```python
from build123d import *

# Parameters (mm, degrees)
EXTRUDE_1_DEPTH = 50


with BuildPart() as part:
    # 草图1 → 凸台-拉伸1 (new body)
    with BuildSketch(Plane.XY):
        with BuildLine():
            Line((-3.068719851, 0.075307347), (-3.068719851, 3.975307347))
            Line((-3.068719851, 3.975307347), (-4.918719851, 3.975307347))
            Line((-4.918719851, 3.975307347), (-4.918719851, 3.125307347))
            Line((-4.918719851, 3.125307347), (-3.918719851, 3.125307347))
            Line((-3.918719851, 3.125307347), (-3.918719851, -3.824692653))
            ThreePointArc((-3.918719851, -3.824692653), (-3.420801379, -5.026774181), (-2.218719851, -5.524692653))
            Line((-2.218719851, -5.524692653), (3.081280149, -5.524692653))
            ThreePointArc((3.081280149, -5.524692653), (4.283361677, -5.026774181), (4.781280149, -3.824692653))
            Line((4.781280149, -3.824692653), (4.781280149, 3.125307347))
            Line((4.781280149, 3.125307347), (5.781280149, 3.125307347))
            Line((5.781280149, 3.125307347), (5.781280149, 3.975307347))
            Line((5.781280149, 3.975307347), (3.931280149, 3.975307347))
            Line((3.931280149, 3.975307347), (3.931280149, 0.075307347))
            Line((3.931280149, 0.075307347), (1.809959806, -2.046012996))
            Line((1.809959806, -2.046012996), (2.110480188, -2.346533378))
            Line((2.110480188, -2.346533378), (3.931280149, -1.126774181))
            Line((3.931280149, -1.126774181), (3.931280149, -3.824692653))
            ThreePointArc((3.931280149, -3.824692653), (3.682320913, -4.425733417), (3.081280149, -4.674692653))
            Line((3.081280149, -4.674692653), (-2.218719851, -4.674692653))
            ThreePointArc((-2.218719851, -4.674692653), (-2.819760615, -4.425733417), (-3.068719851, -3.824692653))
            Line((-3.068719851, -3.824692653), (-3.068719851, -1.126774181))
            Line((-3.068719851, -1.126774181), (-1.247919889, -2.346533378))
            Line((-1.247919889, -2.346533378), (-0.947399507, -2.046012996))
            Line((-0.947399507, -2.046012996), (-3.068719851, 0.075307347))
        make_face()
    extrude(amount=EXTRUDE_1_DEPTH)


solid = part.part
```
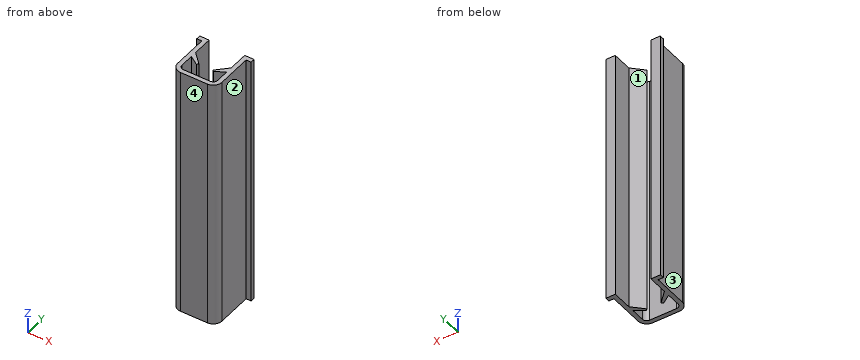
Part model, mm, in its own coordinate system. Face numbers are marked on the shaded views. Round coordinates to 2 decimals unless told otherwise and drop trailing zeros. Write each loop counter-clockwise with the first axis right and the second up, starting at its lowest first coordinate (ties: lowest second). Pieces come first, ordered by that corner, then holes. Notation, with made-up numbers: M 45.25,62 L 76.25,62 A27 ccw 76.25,94 Z; hole C 87.25,36.5 d2. An arc over 180 degrees is marked long. One line per question, with ' | ' between items.
(1) Two-plate mould, pull along X, no slides. Class the marked faces 1, 2, 3 and 4: released by +X, released by -X, zero draft, split by the parting line, or undercut.
Answer key:
face 1: undercut | face 2: released by +X | face 3: released by -X | face 4: zero draft
(2) Probe line 1 along X through (y, z) = (3.25, 38); line 2 along X through (y, z) = (-3.75, 35.5); line 3 along X through (y, z) = (-1.75, 21). List the from-to ranges inside material, lowest first.
Answer key:
line 1: x = -4.92 to -3.07, 3.93 to 5.78 | line 2: x = -3.92 to -3.07, 3.93 to 4.78 | line 3: x = -3.92 to -3.07, -2.14 to -1.24, 2.11 to 3, 3.93 to 4.78
(3) Saw through at A-A on y = 1.5. Write the cut outline in (x, z).
Answer key:
outline: M -3.92,0 L -3.07,0 L -3.07,50 L -3.92,50 Z; M 3.93,0 L 4.78,0 L 4.78,50 L 3.93,50 Z
(4) Saw through at C-C on x = -0.5. Write the cut outline in (y, z), then the cut area to 3 significant figures.
Answer key:
outline: M -5.52,0 L -4.67,0 L -4.67,50 L -5.52,50 Z | area: 42.5 mm^2
(5) Saw through at B-B on z = 23. Write the cut outline in (x, y).
Answer key:
outline: M -4.92,3.13 L -3.92,3.13 L -3.92,-3.82 A1.7 ccw -2.22,-5.52 L 3.08,-5.52 A1.7 ccw 4.78,-3.82 L 4.78,3.13 L 5.78,3.13 L 5.78,3.98 L 3.93,3.98 L 3.93,0.08 L 1.81,-2.05 L 2.11,-2.35 L 3.93,-1.13 L 3.93,-3.82 A0.85 cw 3.08,-4.67 L -2.22,-4.67 A0.85 cw -3.07,-3.82 L -3.07,-1.13 L -1.25,-2.35 L -0.95,-2.05 L -3.07,0.08 L -3.07,3.98 L -4.92,3.98 Z
(6) Pin check, flat tips, straight feed: pin 1 (3 mm diameter, centred on y = 1.5, z = 18.5, fed in from +X); pin 2 (2 mm diameter, centred on y = 1, z = 27, fed in from -X); pin 3 (1 mm diameter, centred on x = 2.5, z = 37, fed in from +Y); pin 4 (1 mm diameter, centred on x = 3.5, y = -3, fed in from +Z). Stop position of each tip, or through.
Answer key:
pin 1: stops at x = 4.78 | pin 2: stops at x = -3.92 | pin 3: stops at y = -0.86 | pin 4: stops at z = 50
